```python
from build123d import *

# Parameters (mm, degrees)
F0_W     = 76.2
F0_H     = 76.2
F1_DEPTH = 3.175
F2_R     = 6.35
F3_DEPTH = 6.35


with BuildPart() as f1:
    # F0 (on Front) → F1 (new body, symmetric)
    with BuildSketch(Plane.XZ):
        with Locations((0, 38.1)):
            Rectangle(F0_W, F0_H)
    extrude(amount=F1_DEPTH, both=True)

    # F2 (on face) → F3 (cut)
    with BuildSketch(Plane.XZ.offset(3.175)):
        with Locations((0, 11.8903209027)):
            Circle(F2_R)
    extrude(amount=-F3_DEPTH, mode=Mode.SUBTRACT)


solid = f1.part
```
Work out the finished part from the listing and answer in its coordinate system (mm). Coordinates: 2 decimals unless noted, no trailing zeros. Order: outer loops, then holes, each group sorted by start corner. A loop starts at its lowest first (then second) coordinate and runs counter-clockwise, first axis right, second up. Notation, with made-up numbers: (77.25, -29) - (128.25, -29) arc R22 cw to (128.25, -21) - close; hole circle Ø7 at (-19.5, 17). An arc over 180 degrees is marked (long way). Answer as a JSON object with one key per item and string values.
1. Consider line 1 (Z direction, x = 0, y = 0.75); line 2 (X direction, y = -0.75, z = 17.5); line 3 (Z direction, x = 4.5, y = -1.5). Determine where each line is inside the solid, lowest interval first.
Output values:
{"line 1": "z = 0 to 5.54, 18.24 to 76.2", "line 2": "x = -38.1 to -2.98, 2.98 to 38.1", "line 3": "z = 0 to 7.41, 16.37 to 76.2"}
2. The mould has two halves that part along X. Classify faces 1 (the face through (-38.1, 0, 38)), 2 (the face through (-1.377, -0.044, 5.691)), 3 (the face through (-1, 3.175, 39)): +X half, -X half, draft (parallel to the pull), parting line (faces both ways), or undercut.
Output values:
{"face 1": "-X half", "face 2": "undercut", "face 3": "draft"}
3. Find section B-B on y = 0. Determine the outline of the cut face in (x, z), plus the area to 3 significant figures.
Output values:
{"outline": "(-38.1, 0) - (38.1, 0) - (38.1, 76.2) - (-38.1, 76.2) - close; hole circle Ø12.7 at (0, 11.89)", "area": "5,680 mm²"}
4. Find section A-A on x = 0. Determine the outline of the cut face in (y, z) (3 decimals).
Output values:
{"outline": "(-3.175, 0) - (3.175, 0) - (3.175, 5.54) - (-3.175, 5.54) - close; (-3.175, 18.24) - (3.175, 18.24) - (3.175, 76.2) - (-3.175, 76.2) - close"}
